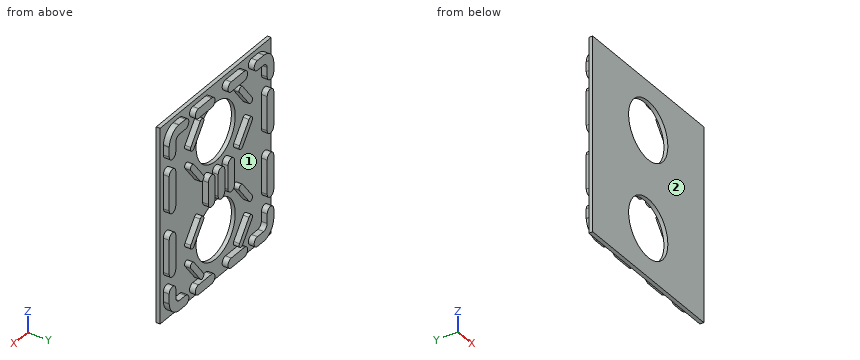
```python
from build123d import *

# Parameters (mm, degrees)
SKETCH1_W               = 170
SKETCH1_H               = 200
BOSS_EXTRUDE1_DEPTH     = 4
BOSS_EXTRUDE2_DEPTH     = 6
CUT_EXTRUDE2_DEPTH      = 263.678510731
CUT_EXTRUDE2_DEPTH_BACK = 10
SKETCH4_R               = 30


with BuildPart() as part:
    # Sketch1 → Boss-Extrude1 (new body)
    with BuildSketch(Plane(origin=(0, 0, 0), x_dir=(1, 0, 0), z_dir=(0, 1, 0))):
        with Locations((85, 100)):
            Rectangle(SKETCH1_W, SKETCH1_H)
    extrude(amount=BOSS_EXTRUDE1_DEPTH)

    # Sketch3 → Boss-Extrude2 (add)
    with BuildSketch(Plane(origin=(0, 4, 0), x_dir=(1, 0, 0), z_dir=(0, 1, 0))):
        with BuildLine():
            Line((30, 15), (20.262068061, 15))
            ThreePointArc((20.262068061, 15), (16.735494747, 16.716132106), (15, 20.233217082))
            Line((15, 20.233217082), (15, 30))
            ThreePointArc((15, 30), (10, 35), (5, 30))
            Line((5, 30), (5, 20))
            Line((5, 20), (4.996202412, 20))
            ThreePointArc((4.996202412, 20), (5.001432837, 19.771358596), (5.017113168, 19.54319555))
            ThreePointArc((5.017113168, 19.54319555), (9.654794827, 9.654664453), (19.545086076, 5.020737673))
            ThreePointArc((19.545086076, 5.020737673), (19.772306824, 5.005187109), (20, 5))
            Line((20, 5), (30, 5))
            ThreePointArc((30, 5), (35, 10), (30, 15))
        make_face()
        with BuildLine():
            Line((5, 85), (5, 50))
            ThreePointArc((5, 50), (10, 45), (15, 50))
            Line((15, 50), (15, 85))
            ThreePointArc((15, 85), (10, 90), (5, 85))
        make_face()
        with BuildLine():
            Line((70, 15), (50, 15))
            ThreePointArc((50, 15), (45, 10), (50, 5))
            Line((50, 5), (70, 5))
            ThreePointArc((70, 5), (75, 10), (70, 15))
        make_face()
        with BuildLine():
            ThreePointArc((155, 50), (160, 45), (165, 50))
            Line((165, 50), (165, 85))
            ThreePointArc((165, 85), (160, 90), (155, 85))
            Line((155, 85), (155, 50))
        make_face()
        with BuildLine():
            ThreePointArc((155, 20.233217082), (153.264505253, 16.716132106), (149.737931939, 15))
            Line((149.737931939, 15), (140, 15))
            ThreePointArc((140, 15), (135, 10), (140, 5))
            Line((140, 5), (150, 5))
            ThreePointArc((150, 5), (150.227693176, 5.005187109), (150.454913924, 5.020737673))
            ThreePointArc((150.454913924, 5.020737673), (160.345205173, 9.654664453), (164.982886832, 19.54319555))
            ThreePointArc((164.982886832, 19.54319555), (165.002074296, 19.868737095), (165, 20.194837008))
            Line((165, 20.194837008), (165, 30))
            ThreePointArc((165, 30), (160, 35), (155, 30))
            Line((155, 30), (155, 20.233217082))
        make_face()
        with BuildLine():
            ThreePointArc((120, 5), (125, 10), (120, 15))
            Line((120, 15), (100, 15))
            ThreePointArc((100, 15), (95, 10), (100, 5))
            Line((100, 5), (120, 5))
        make_face()
        with BuildLine():
            Line((165, 115), (165, 150))
            ThreePointArc((165, 150), (160, 155), (155, 150))
            Line((155, 150), (155, 115))
            ThreePointArc((155, 115), (160, 110), (165, 115))
        make_face()
        with BuildLine():
            Line((155, 179.766782918), (155, 170))
            ThreePointArc((155, 170), (160, 165), (165, 170))
            Line((165, 170), (165, 179.805162992))
            ThreePointArc((165, 179.805162992), (165.002074296, 180.131262905), (164.982886832, 180.45680445))
            ThreePointArc((164.982886832, 180.45680445), (160.345205173, 190.345335547), (150.454913924, 194.979262327))
            ThreePointArc((150.454913924, 194.979262327), (150.227693176, 194.994812891), (150, 195))
            Line((150, 195), (140, 195))
            ThreePointArc((140, 195), (135, 190), (140, 185))
            Line((140, 185), (149.737931939, 185))
            ThreePointArc((149.737931939, 185), (153.264505253, 183.283867894), (155, 179.766782918))
        make_face()
        with BuildLine():
            Line((100, 185), (120, 185))
            ThreePointArc((120, 185), (125, 190), (120, 195))
            Line((120, 195), (100, 195))
            ThreePointArc((100, 195), (95, 190), (100, 185))
        make_face()
        with BuildLine():
            ThreePointArc((50, 195), (45, 190), (50, 185))
            Line((50, 185), (70, 185))
            ThreePointArc((70, 185), (75, 190), (70, 195))
            Line((70, 195), (50, 195))
        make_face()
        with BuildLine():
            ThreePointArc((20, 195), (19.772306824, 194.994812891), (19.545086076, 194.979262327))
            ThreePointArc((19.545086076, 194.979262327), (9.654794827, 190.345335547), (5.017113168, 180.45680445))
            ThreePointArc((5.017113168, 180.45680445), (4.997925704, 180.131262905), (5, 179.805162992))
            Line((5, 179.805162992), (5, 170))
            ThreePointArc((5, 170), (10, 165), (15, 170))
            Line((15, 170), (15, 179.766782918))
            ThreePointArc((15, 179.766782918), (16.735494747, 183.283867894), (20.262068061, 185))
            Line((20.262068061, 185), (30, 185))
            ThreePointArc((30, 185), (35, 190), (30, 195))
            Line((30, 195), (20, 195))
        make_face()
        with BuildLine():
            ThreePointArc((15, 150), (10, 155), (5, 150))
            Line((5, 150), (5, 115))
            ThreePointArc((5, 115), (10, 110), (15, 115))
            Line((15, 115), (15, 150))
        make_face()
        with BuildLine():
            Line((90, 88.83925215), (90, 111.16074785))
            ThreePointArc((90, 111.16074785), (85, 116.16074785), (80, 111.16074785))
            Line((80, 111.16074785), (80, 88.83925215))
            ThreePointArc((80, 88.83925215), (85, 83.83925215), (90, 88.83925215))
        make_face()
        with BuildLine():
            Line((75, 87.963108376), (75, 112.036891624))
            ThreePointArc((75, 112.036891624), (70, 117.036891624), (65, 112.036891624))
            Line((65, 112.036891624), (65, 87.963108376))
            ThreePointArc((65, 87.963108376), (70, 82.963108376), (75, 87.963108376))
        make_face()
        with BuildLine():
            Line((105, 88.843049738), (105, 111.156950262))
            ThreePointArc((105, 111.156950262), (100, 116.156950262), (95, 111.156950262))
            Line((95, 111.156950262), (95, 88.843049738))
            ThreePointArc((95, 88.843049738), (100, 83.843049738), (105, 88.843049738))
        make_face()
        with BuildLine():
            Line((57.382246702, 22.829681435), (42.843957296, 41.823431011))
            ThreePointArc((42.843957296, 41.823431011), (38.638279583, 42.382246702), (38.079463892, 38.176568989))
            Line((38.079463892, 38.176568989), (52.617753298, 19.182819413))
            ThreePointArc((52.617753298, 19.182819413), (56.823431011, 18.624003722), (57.382246702, 22.829681435))
        make_face()
        with BuildLine():
            ThreePointArc((131.920536108, 38.176568989), (131.361720417, 42.382246702), (127.156042704, 41.823431011))
            Line((127.156042704, 41.823431011), (112.617753298, 22.829681435))
            ThreePointArc((112.617753298, 22.829681435), (113.176568989, 18.624003722), (117.382246702, 19.182819413))
            Line((117.382246702, 19.182819413), (131.920536108, 38.176568989))
        make_face()
        with BuildLine():
            Line((112.617753298, 77.170318565), (127.156042704, 58.176568989))
            ThreePointArc((127.156042704, 58.176568989), (131.361720417, 57.617753298), (131.920536108, 61.823431011))
            Line((131.920536108, 61.823431011), (117.382246702, 80.817180587))
            ThreePointArc((117.382246702, 80.817180587), (113.176568989, 81.375996278), (112.617753298, 77.170318565))
        make_face()
        with BuildLine():
            ThreePointArc((38.079463892, 61.823431011), (38.638279583, 57.617753298), (42.843957296, 58.176568989))
            Line((42.843957296, 58.176568989), (57.382246702, 77.170318565))
            ThreePointArc((57.382246702, 77.170318565), (56.823431011, 81.375996278), (52.617753298, 80.817180587))
            Line((52.617753298, 80.817180587), (38.079463892, 61.823431011))
        make_face()
        with BuildLine():
            ThreePointArc((38.079463892, 161.823431011), (38.638279583, 157.617753298), (42.843957296, 158.176568989))
            Line((42.843957296, 158.176568989), (57.382246702, 177.170318565))
            ThreePointArc((57.382246702, 177.170318565), (56.823431011, 181.375996278), (52.617753298, 180.817180587))
            Line((52.617753298, 180.817180587), (38.079463892, 161.823431011))
        make_face()
        with BuildLine():
            Line((112.617753298, 177.170318565), (127.156042704, 158.176568989))
            ThreePointArc((127.156042704, 158.176568989), (131.361720417, 157.617753298), (131.920536108, 161.823431011))
            Line((131.920536108, 161.823431011), (117.382246702, 180.817180587))
            ThreePointArc((117.382246702, 180.817180587), (113.176568989, 181.375996278), (112.617753298, 177.170318565))
        make_face()
        with BuildLine():
            ThreePointArc((131.920536108, 138.176568989), (131.361720417, 142.382246702), (127.156042704, 141.823431011))
            Line((127.156042704, 141.823431011), (112.617753298, 122.829681435))
            ThreePointArc((112.617753298, 122.829681435), (113.176568989, 118.624003722), (117.382246702, 119.182819413))
            Line((117.382246702, 119.182819413), (131.920536108, 138.176568989))
        make_face()
        with BuildLine():
            Line((57.382246702, 122.829681435), (42.843957296, 141.823431011))
            ThreePointArc((42.843957296, 141.823431011), (38.638279583, 142.382246702), (38.079463892, 138.176568989))
            Line((38.079463892, 138.176568989), (52.617753298, 119.182819413))
            ThreePointArc((52.617753298, 119.182819413), (56.823431011, 118.624003722), (57.382246702, 122.829681435))
        make_face()
    extrude(amount=BOSS_EXTRUDE2_DEPTH)

    # Sketch4 → Cut-Extrude2 (cut, two sides: drawn at the far end of the back side and taken through both)
    with BuildSketch(Plane(origin=(0, 0, 0), x_dir=(1, 0, 0), z_dir=(0, 1, 0)).offset(-CUT_EXTRUDE2_DEPTH_BACK)):
        with Locations(Location((85, 50, 0), (0, 0, 90))):
            Circle(SKETCH4_R)
        with Locations(Location((85, 150, 0), (0, 0, 90))):
            Circle(SKETCH4_R)
    extrude(amount=CUT_EXTRUDE2_DEPTH + CUT_EXTRUDE2_DEPTH_BACK, mode=Mode.SUBTRACT)


solid = part.part
```
Build history of the part. All positions in model axes, mm. Face numbers are marked on the shaded views. Coordinates: 2 decimals unless noted, no trailing zeros. Order: outer loops, then holes, each group sorted by start corner. A loop starts at its lowest first (then second) coordinate and runs counter-clockwise, first axis right, second up. Notation, with made-up numbers: M -30.75,4.5 L -3.75,4.5 A29 ccw -3.75,24.5 Z; hole C 37.25,-31.75 d2. An arc over 180 degrees is marked long. One line per question, with ' | ' between items. Start each with the question number.
1. Cut at C-C (y = 8.5). Count the separate pieces of the cut face and the enclosed holes in it, plus the area to 3 significant figures.
2. Flat gauge pins, fed straight in: P1, Ø3, axis at y = 6, z = -101, coming from the -X side; P2, Ø4, axis at y = 7, z = -141, coming from the -X side; P3, Ø1.8, axis at y = 7, z = -102, coming from the +X side; P4, Ø1.5, axis at y = 1.5, z = -115, coming from the -X side. Where does each tip first touch, or does it go through?
3. Mould opens along X. For the marked faces 1 and 2 say: +X half, -X half, draft (parallel to the pull), parting line (faces both ways), or undercut.
4. Wall check: line 1 along Z through (x, y) = (20, 8.25); line 2 along Z through (x, y) = (121.5, 5); line 3 along X through (y, z) = (8.5, -55). Give the ranges that are in metal, low to high. Write a range as [from, to].
5. Cut at A-A (x = 92.5). Write the cut outline in (y, z), plus the area to 3 significant figures.
6. Cut at B-B (z = -126.5). Write the cut outline in (x, y), plus the area to 3 significant figures.
7. Cut at D-D (x = 160). Write the cut outline in (y, z), plus the area to 3 significant figures.
The answers:
1) separate pieces: 23 | enclosed holes: 0 | area: 6,850 mm2
2) P1: stops at x = 65 | P2: stops at x = 5 | P3: stops at x = 105 | P4: stops at x = 0
3) face 1: undercut | face 2: draft
4) line 1: z = [-195, -184.96], [-15.04, -5] | line 2: z = [-194.77, -185.23], [-175.44, -165.57], [-134.43, -124.56], [-75.44, -65.57], [-34.43, -24.56], [-14.77, -5.23] | line 3: x = [5, 15], [155, 165]
5) outline: M 0,-200 L 4,-200 L 4,-179.05 L 0,-179.05 Z; M 0,-120.95 L 4,-120.95 L 4,-79.05 L 0,-79.05 Z; M 0,-20.95 L 4,-20.95 L 4,0 L 0,0 Z | area: 335 mm2
6) outline: M 0,0 L 66.35,0 L 66.35,4 L 54.57,4 L 54.57,10 L 47.02,10 L 47.02,4 L 15,4 L 15,10 L 5,10 L 5,4 L 0,4 Z; M 103.65,0 L 170,0 L 170,4 L 165,4 L 165,10 L 155,10 L 155,4 L 122.98,4 L 122.98,10 L 115.43,10 L 115.43,4 L 103.65,4 Z | area: 741 mm2
7) outline: M 0,-200 L 4,-200 L 4,-190.68 L 10,-190.68 L 10,-165 L 4,-165 L 4,-155 L 10,-155 L 10,-110 L 4,-110 L 4,-90 L 10,-90 L 10,-45 L 4,-45 L 4,-35 L 10,-35 L 10,-9.32 L 4,-9.32 L 4,0 L 0,0 Z | area: 1,650 mm2
